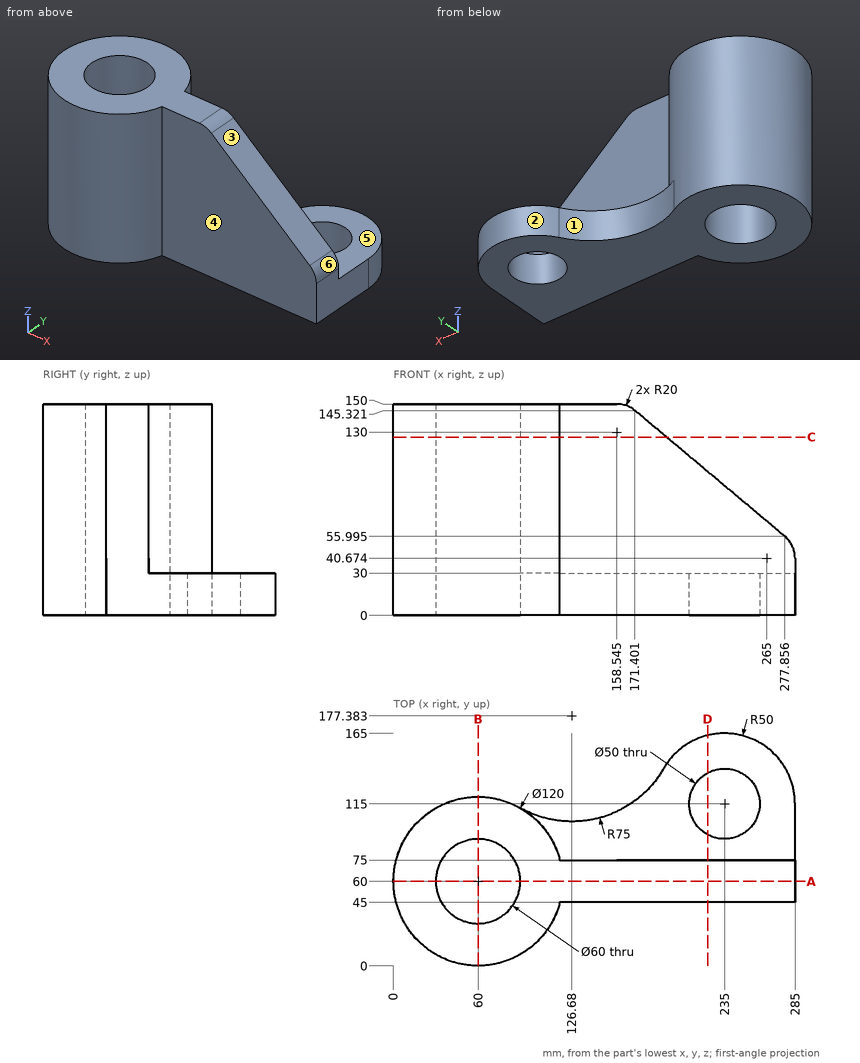
The drawing under review shows one solid part. Ordinate dimensions are in mm from its lowest x, y, z. A direction names the side the tool comes from. Give positions to 0.01 mm unless a question says otherwise; leave off trailing zeros. Order: outer loops, then holes, each group sorted by start corner. A loop starts at its lowest first (then second) coordinate and runs counter-clockwise, first axis right, second up. Notation, with made-up numbers: (-39.5, 83) - (-32.5, 83) arc R25 cw to (-32.5, 113) - close; hole circle Ø2 at (10.5, -1). An arc over 180 degrees is marked (long way). Answer as a JSON object with one key per item and string values. Group by question number.
Item 1: Take a section at B-B on x = 60. Give the boundary of the cut face in (y, z), and give its area (3 significant figures).
Item 2: Clearance check with flat-ended pins moving along their axes: pin 1 Ø1.5 at (x, z) = (91, 96.5) entering from -Y; pin 2 Ø4 at (x, z) = (211.5, 105) entering from -Y; pin 3 Ø1.5 at (y, z) = (71, 105) entering from -X. State where each tip first meets the part, or that it passes through.
Item 3: Draft analysis for pull direction X (two halves, no side actions). For the marked faces 1, 2 and 3, state which applies: pulls with the +X half, pulls with the -X half, needs draft (parallel to the pull), parting line crosses it, or undercut.
Item 4: Take a section at C-C on z = 126.5. Give the boundary of the cut face in (x, y) (1 decimal).
Item 5: Take a section at A-A on y = 60. Give the boundary of the cut face in (x, z) (1 decimal), and give its area (3 significant figures).
Item 6: Wall thickness on line 1 along Y through (x, z) = (60, 72); line 2 along Y through (x, z) = (235, 16.75); line 3 along X through (y, z) = (115, 13) (1 decimal): over which ranges is each line inside the solid? List them lowest first.
Item 7: Take a section at D-D on x = 223. Give the boundary of the cut face in (y, z) (1 decimal), and give its area (3 significant figures).
Item 8: Machinability: for the marked faces 4, 5 and 6, which of the approach directions +Z, -Z, +X, -X, +Y, -Y give a long, thin tool a straight path to every point of the face, cutting with its end or side? Answer none if there is none.
Reported:
{
 "1": {"outline": "(0, 0) - (30, 0) - (30, 150) - (0, 150) - close; (90, 0) - (120, 0) - (120, 150) - (90, 150) - close", "area": "9,000 mm^2"},
 "2": {"pin 1": "y = 8.18", "pin 2": "y = 45", "pin 3": "x = 0.88"},
 "3": {"face 1": "undercut", "face 2": "parting line crosses it", "face 3": "pulls with the +X half"},
 "4": {"outline": "(118.1, 45) - (193.8, 45) - (193.8, 75) - (118.1, 75) arc R60 ccw (long way) to start; hole circle Ø60 at (60, 60)"},
 "5": {"outline": "(0, 0) - (30, 0) - (30, 150) - (0, 150) - close; (90, 0) - (285, 0) - (285, 40.7) arc R20 ccw to (277.9, 56) - (171.4, 145.3) arc R20 ccw to (158.5, 150) - (90, 150) - close", "area": "27,800 mm^2"},
 "6": {"line 1": "0 to 30, 90 to 120", "line 2": "45 to 90, 140 to 165", "line 3": "36 to 84, 168.3 to 210, 260 to 285"},
 "7": {"outline": "(45, 0) - (93.1, 0) - (93.1, 30) - (75, 30) - (75, 102) - (45, 102) - close; (136.9, 0) - (163.5, 0) - (163.5, 30) - (136.9, 30) - close", "area": "4,400 mm^2"},
 "8": {"face 4": "+Z, -Z, +X, -Y", "face 5": "+Z, +X, +Y", "face 6": "+Z, +X, +Y, -Y"}
}
